```python
from build123d import *

# Parameters (mm, degrees)
SKETCH1_W                    = 15
SKETCH1_H                    = 15
BOSS_EXTRUDE1_DEPTH          = 3.175
SKETCH2_W                    = 2.75
SKETCH2_H                    = 2.5
SKETCH2_H_2                  = 4
SKETCH2_W_2                  = 1.125
SKETCH2_H_3                  = 7.5
CUT_EXTRUDE1_DEPTH           = 141.379634965
CIRPATTERN1_COUNT            = 4
F_3_0_3_DIAMETER_HOLE1_D     = 3
F_8_0_8_DIAMETER_HOLE1_D     = 8
F_8_0_8_DIAMETER_HOLE1_DEPTH = 6.35


with BuildPart() as part:
    # Sketch1 → Boss-Extrude1 (new, symmetric)
    with BuildSketch(Plane(origin=(0, 0, 0), x_dir=(1, 0, 0), z_dir=(0, 1, 0))):
        with BuildLine():
            Line((-83.903460262, -7.5), (-98.95418457, -7.5))
            ThreePointArc((-98.95418457, -7.5), (-70.171862751, -70.171862751), (-7.5, -98.95418457))
            Line((-7.5, -98.95418457), (-7.5, -83.903460262))
            ThreePointArc((-7.5, -83.903460262), (-59.565261034, -59.565261034), (-83.903460262, -7.5))
        make_face()
        with BuildLine():
            ThreePointArc((-98.95418457, 7.5), (-99.238, 0), (-98.95418457, -7.5))
            Line((-98.95418457, -7.5), (-83.903460262, -7.5))
            ThreePointArc((-83.903460262, -7.5), (-84.238, 0), (-83.903460262, 7.5))
            Line((-83.903460262, 7.5), (-98.95418457, 7.5))
        make_face()
        with BuildLine():
            Line((83.903460262, -7.5), (98.95418457, -7.5))
            ThreePointArc((98.95418457, -7.5), (99.167020759, -3.752684079), (99.238, 0))
            ThreePointArc((99.238, 0), (99.167020759, 3.752684079), (98.95418457, 7.5))
            Line((98.95418457, 7.5), (83.903460262, 7.5))
            ThreePointArc((83.903460262, 7.5), (84.154323506, 3.753728707), (84.238, 0))
            ThreePointArc((84.238, 0), (84.154323506, -3.753728707), (83.903460262, -7.5))
        make_face()
        with BuildLine():
            ThreePointArc((-7.5, 98.95418457), (-70.171862751, 70.171862751), (-98.95418457, 7.5))
            Line((-98.95418457, 7.5), (-83.903460262, 7.5))
            ThreePointArc((-83.903460262, 7.5), (-59.565261034, 59.565261034), (-7.5, 83.903460262))
            Line((-7.5, 83.903460262), (-7.5, 98.95418457))
        make_face()
        with BuildLine():
            Line((-7.5, -83.903460262), (-7.5, -98.95418457))
            ThreePointArc((-7.5, -98.95418457), (0, -99.238), (7.5, -98.95418457))
            Line((7.5, -98.95418457), (7.5, -83.903460262))
            ThreePointArc((7.5, -83.903460262), (0, -84.238), (-7.5, -83.903460262))
        make_face()
        with BuildLine():
            ThreePointArc((7.5, 98.95418457), (0, 99.238), (-7.5, 98.95418457))
            Line((-7.5, 98.95418457), (-7.5, 83.903460262))
            ThreePointArc((-7.5, 83.903460262), (0, 84.238), (7.5, 83.903460262))
            Line((7.5, 83.903460262), (7.5, 98.95418457))
        make_face()
        with BuildLine():
            ThreePointArc((98.95418457, 7.5), (70.171862751, 70.171862751), (7.5, 98.95418457))
            Line((7.5, 98.95418457), (7.5, 83.903460262))
            ThreePointArc((7.5, 83.903460262), (59.565261034, 59.565261034), (83.903460262, 7.5))
            Line((83.903460262, 7.5), (98.95418457, 7.5))
        make_face()
        with BuildLine():
            Line((7.5, -83.903460262), (7.5, -98.95418457))
            ThreePointArc((7.5, -98.95418457), (70.171862751, -70.171862751), (98.95418457, -7.5))
            Line((98.95418457, -7.5), (83.903460262, -7.5))
            ThreePointArc((83.903460262, -7.5), (59.565261034, -59.565261034), (7.5, -83.903460262))
        make_face()
        with BuildLine():
            Line((7.5, -7.5), (-7.5, -7.5))
            Line((-7.5, -7.5), (-7.5, -83.903460262))
            ThreePointArc((-7.5, -83.903460262), (0, -84.238), (7.5, -83.903460262))
            Line((7.5, -83.903460262), (7.5, -7.5))
        make_face()
        with BuildLine():
            ThreePointArc((-83.903460262, 7.5), (-84.238, 0), (-83.903460262, -7.5))
            Line((-83.903460262, -7.5), (-7.5, -7.5))
            Line((-7.5, -7.5), (-7.5, 7.5))
            Line((-7.5, 7.5), (-83.903460262, 7.5))
        make_face()
        with BuildLine():
            Line((-7.5, 83.903460262), (-7.5, 7.5))
            Line((-7.5, 7.5), (7.5, 7.5))
            Line((7.5, 7.5), (7.5, 83.903460262))
            ThreePointArc((7.5, 83.903460262), (0, 84.238), (-7.5, 83.903460262))
        make_face()
        with BuildLine():
            Line((7.5, 7.5), (7.5, -7.5))
            Line((7.5, -7.5), (83.903460262, -7.5))
            ThreePointArc((83.903460262, -7.5), (84.154323506, -3.753728707), (84.238, 0))
            ThreePointArc((84.238, 0), (84.154323506, 3.753728707), (83.903460262, 7.5))
            Line((83.903460262, 7.5), (7.5, 7.5))
        make_face()
        Rectangle(SKETCH1_W, SKETCH1_H)
    extrude(amount=BOSS_EXTRUDE1_DEPTH, both=True)

    # Sketch2 → Cut-Extrude1 (cut, symmetric)
    with BuildSketch(Plane(origin=(0, 0, 0), x_dir=(1, 0, 0), z_dir=(0, 1, 0))):
        with Locations((0, 86.488)):
            Rectangle(SKETCH2_W, SKETCH2_H)
        with Locations((0, 89.738)):
            Rectangle(SKETCH2_W, SKETCH2_H_2)
        with Locations((1.9375, 89.738)):
            Rectangle(SKETCH2_W_2, SKETCH2_H_2)
        with Locations((0, 95.488)):
            Rectangle(SKETCH2_W, SKETCH2_H_3)
        with Locations((-1.9375, 89.738)):
            Rectangle(SKETCH2_W_2, SKETCH2_H_2)
    cut_extrude1 = extrude(amount=CUT_EXTRUDE1_DEPTH, both=True, mode=Mode.SUBTRACT)

    # CirPattern1: Cut-Extrude1 ×4 about axis
    cirpattern1_axis = Axis((0, 0, 0), (0, 1, 0))
    for i in range(1, CIRPATTERN1_COUNT):
        add(cut_extrude1.rotate(cirpattern1_axis, i * 360 / CIRPATTERN1_COUNT), mode=Mode.SUBTRACT)

    # Ø3.0 (3) Diameter Hole1 (through all)
    with Locations(Plane(origin=(0, 3.175, 0), x_dir=(1, 0, 0), z_dir=(0, 1, 0))):
        with Locations((-64.868561892, -64.868561892), (0, 0), (-64.868561892, 64.868561892), (64.868561892, 64.868561892), (64.868561892, -64.868561892)):
            Hole(F_3_0_3_DIAMETER_HOLE1_D / 2)

    # Ø8.0 (8) Diameter Hole1
    with Locations(Plane(origin=(0, 3.175, 0), x_dir=(1, 0, 0), z_dir=(0, 1, 0))):
        with Locations((0, 0)):
            Hole(F_8_0_8_DIAMETER_HOLE1_D / 2, depth=F_8_0_8_DIAMETER_HOLE1_DEPTH)


solid = part.part
```
The model under review builds one solid part; all positions refer to its coordinate system, in mm. A direction names the side the tool comes from. Round coordinates to 2 decimals unless told otherwise and drop trailing zeros. Loops run counter-clockwise (first coordinate to the right, second up) from the corner with the lowest first, then second, coordinate; pieces in that order, holes last. Notation, with made-up numbers: (28, 48) -> (58, 48) arc R34 ccw to (58, 83) -> close; hole circle Ø2 at (-27.75, -19.5). An arc over 180 degrees is marked (long way). Answer as a JSON object with one key per item and string values. Group by question number.
1) We need section B-B on z = 45.5. Write out the cut boundary in (x, y) (3 decimals), then the cut area to 3 significant figures.
2) We need section A-A on x = 61. Write out the cut boundary in (y, z) (3 decimals).
3) For line 1 (Z direction, x = 0, y = 0); line 2 (X direction, y = 2.25, z = -54); line 3 (Z direction, x = -60, y = 1.25), list the stretches that pass through material, from the lowest coordinate up. Write a range as [from, to].
4) Mouldability with a two-part tool opening along Z and no side actions: class faces 1 (the face through (95, 0, 1.375)), 2 (the face through (1.375, 0, 96)) as released by +Z, released by -Z, zero draft, split by the parting line, or undercut.
5) For faces 3 (the face through (7.5, 0, -45)), 4 (the face through (0, -3.175, 7)), 5 (the face through (1.375, 0, -95)), 6 (the face through (-96, 0, 1.375)), 7 (the face through (96, 0, -1.375)), list the 3-axis set-ups (+Z, -Z, +X, -X, +Y, -Y) from which the entire face can be reached by the end or side of a thin tool; tool diameter is ignored.
6) We need section C-C on y = -2. Give the number of separate pieces and of enclosed holes in the cut face, then the cut area to 3 significant figures.
7) For pin 1 Ø0.9 at (x, y) = (2, -1.5) entering from +Z; pin 2 Ø1.4 at (x, y) = (-0.5, -1.5) entering from -Z; pin 3 Ø2 at (y, z) = (0, 89) entering from -X; pin 4 Ø3.5 at (x, z) = (-64.87, 64.87) entering from +Y (3 decimals), all flat-tipped, find the tip position at first contact; note any pin that passes through.
Result set:
{
 "1": {"outline": "(-88.193, -3.175) -> (-70.893, -3.175) -> (-70.893, 3.175) -> (-88.193, 3.175) -> close; (-7.5, -3.175) -> (7.5, -3.175) -> (7.5, 3.175) -> (-7.5, 3.175) -> close; (70.893, -3.175) -> (88.193, -3.175) -> (88.193, 3.175) -> (70.893, 3.175) -> close", "area": "315 mm²"},
 "2": {"outline": "(-3.175, -78.276) -> (3.175, -78.276) -> (3.175, -58.095) -> (-3.175, -58.095) -> close; (-3.175, -7.5) -> (3.175, -7.5) -> (3.175, 7.5) -> (-3.175, 7.5) -> close; (-3.175, 58.095) -> (3.175, 58.095) -> (3.175, 78.276) -> (-3.175, 78.276) -> close"},
 "3": {"line 1": "[-85.24, -4], [4, 85.24]", "line 2": "[-83.26, -64.65], [-7.5, 7.5], [64.65, 83.26]", "line 3": "[-79.05, -59.13], [-7.5, 7.5], [59.13, 79.05]"},
 "4": {"face 1": "undercut", "face 2": "zero draft"},
 "5": {"face 3": "+Y, -Y", "face 4": "+Z, -Z, +X, -X, -Y", "face 5": "-Z, +Y, -Y", "face 6": "-X, +Y, -Y", "face 7": "+X, +Y, -Y"},
 "6": {"separate pieces": "1", "enclosed holes": "9", "area": "13,200 mm²"},
 "7": {"pin 1": "z = 99.23", "pin 2": "z = -85.24", "pin 3": "x = -45.87", "pin 4": "y = 3.175"}
}
